Geometry: final body of the model. Coordinates: model frame, mm. Face numbers are marked on the shaded views. A direction names the side the tool comes from. Coordinates: 2 decimals unless noted, no trailing zeros. Loops run counter-clockwise (first coordinate to the right, second up) from the corner with the lowest first, then second, coordinate; pieces in that order, holes last. Notation, with made-up numbers: (24, 22.5) - (32, 22.5) arc R14 cw to (32, 45.5) - close; hole circle Ø10 at (84.25, 52). An arc over 180 degrees is marked (long way). Put each result on its own line as item: value. Start each with the question number.
1) Contact query for flat-ended pins moving along their axis: pin 1 Ø1 at (y, z) = (4.5, 17.5) entering from +X; pin 2 Ø1.8 at (x, y) = (-15.5, 28.5) entering from -Z; pin 3 Ø19 at (x, z) = (-9.5, 28.5) entering from -Y; pin 4 Ø1.5 at (x, y) = (-0.5, 27) entering from -Z. Output: stop coordinate, or through.
2) Draft query along X for the marked faces 3, 4 and 5. Return one class per face: +X half, -X half, draft (parallel to the pull), parting line (faces both ways), or undercut.
3) Section B-B on z = 43. Count the separate pieces of the cut face and the enclosed holes in it, and give its area (3 significant figures).
4) Material intervals for line 1 along Y through (x, z) = (29, 2.9); line 2 along X through (y, z) = (-19, 1.8); line 3 along X through (y, z) = (27, 46.5), sorted ascending. Write a range as from..to.
5) Section A-A on x = -13. Output: boundary loops of the cut face in (y, z).
6) Reachability of the marked faces 1 and 2 from +Z, -Z, +X, -X, +Y, -Y: full face, straight path, thin tool, end or side. Return the list, or none.
```python
from build123d import *

# Parameters (mm, degrees)
SKETCH1_W                      = 70
SKETCH1_H                      = 50
BOSS_EXTRUDE1_DEPTH            = 4
BOSS_EXTRUDE2_DEPTH            = 52
CUT_EXTRUDE3_DEPTH             = 70.491006612
CUT_EXTRUDE3_DEPTH_BACK        = 70.491006612
FILLET1_R                      = 6
CUT_EXTRUDE6_DEPTH             = 84.390646958
SKETCH7_W                      = 22
SKETCH7_H                      = 9
CUT_EXTRUDE7_DEPTH             = 67.550732528
F_4_2_4_2_DIAMETER_HOLE1_D     = 4.2
F_4_2_4_2_DIAMETER_HOLE1_DEPTH = 4
F_4_2_4_2_DIAMETER_HOLE1_TIP   = 1.2618073
CUT_EXTRUDE8_REACH             = 68.551
BOSS_EXTRUDE3_DEPTH            = 6
FILLET2_R                      = 2
FILLET3_R                      = 1
FILLET4_R                      = 1


with BuildPart() as part:
    # Sketch1 → Boss-Extrude1 (new body)
    with BuildSketch(Plane.XY):
        Rectangle(SKETCH1_W, SKETCH1_H)
    extrude(amount=BOSS_EXTRUDE1_DEPTH)

    # Sketch2 → Boss-Extrude2 (add)
    with BuildSketch(Plane.XY):
        Polygon((-23, -25), (-20, -25), (-20, 24), (-11, 24), (-11, 30), (-23, 30), align=None)
        Polygon((11, 24), (11, 30), (23, 30), (23, -25), (20, -25), (20, 24), align=None)
    extrude(amount=BOSS_EXTRUDE2_DEPTH)

    # Sketch3 → Cut-Extrude3 (cut, two sides: drawn at the far end of the back side and taken through both)
    with BuildSketch(Plane.ZY.offset(-CUT_EXTRUDE3_DEPTH_BACK)):
        Polygon((178.049174714, 101.910856562), (52, 10), (4, -25), (-122.049174714, -116.910856562), (61.77253841, -369.00920599), (361.870887838, -150.187492865), align=None)
    extrude(amount=CUT_EXTRUDE3_DEPTH + CUT_EXTRUDE3_DEPTH_BACK, mode=Mode.SUBTRACT)

    # Fillet1
    fillet1_edges = [part.edges().sort_by_distance(p)[0] for p in [
        (35, -25, 2),
        (-35, -25, 2),
        (-35, 25, 2),
        (35, 25, 2),
    ]]
    fillet(fillet1_edges, radius=FILLET1_R)

    # Sketch6 → Cut-Extrude6 (cut, through all)
    with BuildSketch(Plane(origin=(0, 30, 0), x_dir=(1, 0, 0), z_dir=(0, 1, 0))):
        Polygon((-17.1, -47.114359354), (-17.1, -39.885640646), (-16.3, -38.5), (-14.7, -38.5), (-13.9, -39.885640646), (-13.9, -47.114359354), (-14.7, -48.5), (-16.3, -48.5), align=None)
        Polygon((16.3, -48.5), (17.1, -47.114359354), (17.1, -39.885640646), (16.3, -38.5), (14.7, -38.5), (13.9, -39.885640646), (13.9, -47.114359354), (14.7, -48.5), align=None)
        Polygon((17.1, -8.885640646), (17.1, -16.114359354), (16.3, -17.5), (14.7, -17.5), (13.9, -16.114359354), (13.9, -8.885640646), (14.7, -7.5), (16.3, -7.5), align=None)
        Polygon((-16.3, -7.5), (-17.1, -8.885640646), (-17.1, -16.114359354), (-16.3, -17.5), (-14.7, -17.5), (-13.9, -16.114359354), (-13.9, -8.885640646), (-14.7, -7.5), align=None)
    extrude(amount=-CUT_EXTRUDE6_DEPTH, mode=Mode.SUBTRACT)

    # Sketch7 → Cut-Extrude7 (cut, through all)
    with BuildSketch(Plane.XY.offset(4)):
        with Locations((0, 20.5)):
            Rectangle(SKETCH7_W, SKETCH7_H)
    extrude(amount=-CUT_EXTRUDE7_DEPTH, mode=Mode.SUBTRACT)

    # Ø4.2 (4.2) Diameter Hole1
    with Locations(Plane.XY.offset(4)):
        with Locations((-29, -19), (-29, 11), (29, -19), (29, 11)):
            Hole(F_4_2_4_2_DIAMETER_HOLE1_D / 2, depth=F_4_2_4_2_DIAMETER_HOLE1_DEPTH)
            with Locations((0, 0, -(F_4_2_4_2_DIAMETER_HOLE1_DEPTH + F_4_2_4_2_DIAMETER_HOLE1_TIP / 2))):  # 118° drill point
                Cone(0, F_4_2_4_2_DIAMETER_HOLE1_D / 2, F_4_2_4_2_DIAMETER_HOLE1_TIP, mode=Mode.SUBTRACT)

    # Sketch10 → Cut-Extrude8 (cut, up to next)
    with BuildSketch(Plane.XY.offset(4), mode=Mode.PRIVATE) as cut_extrude8_sk1:
        with BuildLine():
            Line((1.414213562, 5.899494937), (9.899494937, -2.585786438))
            ThreePointArc((9.899494937, -2.585786438), (10.485281374, -4), (9.899494937, -5.414213562))
            Line((9.899494937, -5.414213562), (1.414213562, -13.899494937))
            ThreePointArc((1.414213562, -13.899494937), (0, -14.485281374), (-1.414213562, -13.899494937))
            Line((-1.414213562, -13.899494937), (-9.899494937, -5.414213562))
            ThreePointArc((-9.899494937, -5.414213562), (-10.485281374, -4), (-9.899494937, -2.585786438))
            Line((-9.899494937, -2.585786438), (-1.414213562, 5.899494937))
            ThreePointArc((-1.414213562, 5.899494937), (0, 6.485281374), (1.414213562, 5.899494937))
        make_face()
    cut_extrude8_tool1 = extrude(cut_extrude8_sk1.sketch, amount=-CUT_EXTRUDE8_REACH, mode=Mode.PRIVATE) & part.part
    add(cut_extrude8_tool1.solids().sort_by_distance((0, -4, 4))[0], mode=Mode.SUBTRACT)

    # Sketch11 → Boss-Extrude3 (add)
    with BuildSketch(Plane(origin=(0, 30, 0), x_dir=(1, 0, 0), z_dir=(0, 1, 0))):
        with BuildLine():
            Line((-1.5, -46.056349186), (-7.778174593, -39.778174593))
            ThreePointArc((-7.778174593, -39.778174593), (-10.162674858, -36.209517756), (-11, -32))
            Line((-11, -32), (-11, -52))
            Line((-11, -52), (11, -52))
            Line((11, -52), (11, -32))
            ThreePointArc((11, -32), (10.162674858, -36.209517756), (7.778174593, -39.778174593))
            Line((7.778174593, -39.778174593), (1.5, -46.056349186))
            Line((1.5, -46.056349186), (-1.5, -46.056349186))
        make_face()
    extrude(amount=-BOSS_EXTRUDE3_DEPTH)

    # Fillet2
    fillet2_edges = [part.edges().sort_by_distance(p)[0] for p in [
        (-23, 25, 2),
        (-23, 30, 26),
        (-11, 16, 2),
        (11, 16, 2),
        (23, 25, 2),
        (23, 30, 26),
    ]]
    fillet(fillet2_edges, radius=FILLET2_R)

    # Fillet3
    fillet3_edges = [part.edges().sort_by_distance(p)[0] for p in [
        (11, 30, 16),
        (-11, 30, 16),
        (-10.162674858, 30, 36.209517756),
        (10.162674858, 30, 36.209517756),
        (4.639087297, 30, 42.91726189),
        (0, 30, 46.056349186),
        (-4.639087297, 30, 42.91726189),
    ]]
    fillet(fillet3_edges, radius=FILLET3_R)

    # Fillet4
    fillet4_edges = [part.edges().sort_by_distance(p)[0] for p in [
        (-20, 24, 28),
        (11, 24, 18),
        (-11, 24, 18),
        (-10.162674858, 24, 36.209517756),
        (-4.639087297, 24, 42.91726189),
        (0, 24, 46.056349186),
        (4.639087297, 24, 42.91726189),
        (10.162674858, 24, 36.209517756),
        (20, 24, 28),
        (-23, -7.5, 28),
        (-20, -7.5, 28),
        (20, -7.5, 28),
        (23, -7.5, 28),
    ]]
    fillet(fillet4_edges, radius=FILLET4_R)


solid = part.part
```
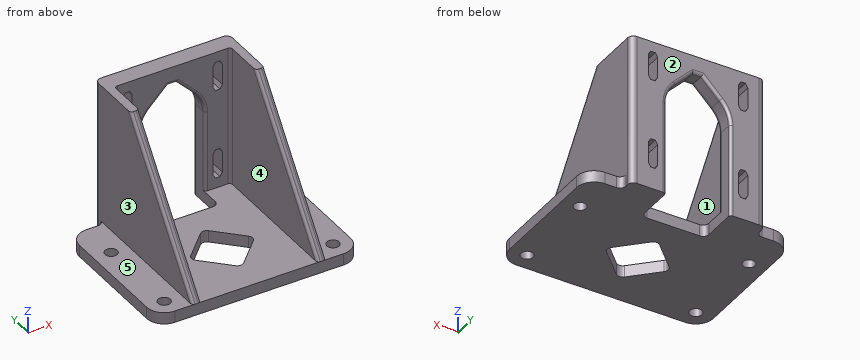
Answer block:
1. pin 1: stops at x = 23
1. pin 2: stops at z = 0
1. pin 3: stops at y = 24
1. pin 4: stops at z = 46.06
2. face 3: -X half
2. face 4: undercut
2. face 5: draft
3. separate pieces: 4
3. enclosed holes: 0
3. area: 303 mm²
4. line 1: y = -25..-21.1, -16.9..8.9, 13.1..25
4. line 2: x = -35..-31.1, -26.9..26.9, 31.1..35
4. line 3: x = -23..-17.1, -13.9..13.9, 17.1..23
5. outline: (-25, 0) - (30, 0) - (30, 52) - (24, 52) - (24, 4) - (-25, 4) - close
6. face 1: +Z, -Y
6. face 2: +Z, -Z, +X, -X, +Y
